CAD build for the part. Positions are in the model's coordinates, mm. Round coordinates to 2 decimals unless told otherwise and drop trailing zeros. Loops run counter-clockwise (first coordinate to the right, second up) from the corner with the lowest first, then second, coordinate; pieces in that order, holes last. Notation, with made-up numbers: M -35.5,78.5 L -10.5,78.5 A24 ccw -10.5,89.5 Z; hole C 83.5,-9.75 d3. An arc over 180 degrees is marked long. One line per item, written item: value. Start each with the question number.
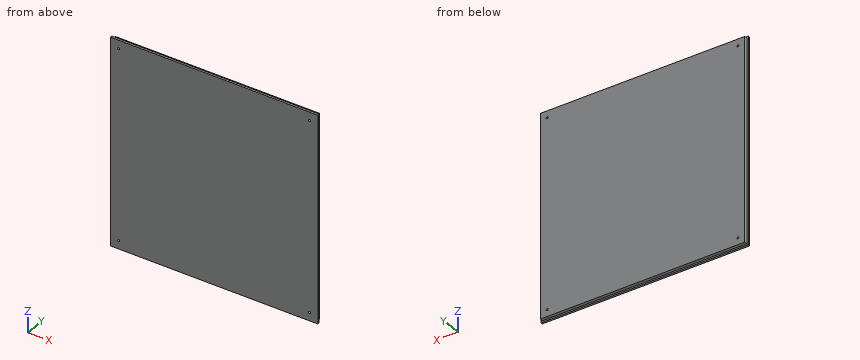
Autodesk Inventor part; units mm, degrees
ref_plane "YZ Plane" through (0, 0, 0) normal (1, 0, 0) x (0, 1, 0)
ref_plane "XZ Plane" through (0, 0, 0) normal (0, 1, 0) x (-1, 0, 0)
ref_plane "XY Plane" through (0, 0, 0) normal (0, 0, 1) x (1, 0, 0)
sketch "Boceto1" plane through (0, 0, 0) normal (0, 1, 0) x (-1, 0, 0)
  line L0 (-103, 103) -> (103, 103)
  line L1 (103, 103) -> (103, -103)
  line L2 (103, -103) -> (-103, -103)
  line L3 (-103, -103) -> (-103, 103)
  line L4 (-103, 103) -> (103, -103) construction
  line L5 (103, 103) -> (-103, -103) construction
  point P0 (0, 0)
  dimension "d0" = 206
  dimension "d1" = 206
extrude "Extrusión1" add sketch "Boceto1" along normal blind 5
sketch "Boceto3" plane through (0, 5, 0) normal (0, 1, 0) x (1, 0, 0)
  line L0 (85, 100) -> (103, 100)
  line L1 (103, -103) -> (103, 103)
  line L2 (100, -85) -> (100, 85)
  line L3 (100, 85) -> (100, 100)
  line L4 (100, 100) -> (116.202, 100) construction
  arc A0 (85, 100) -> (100, 85) centre (100, 100) ccw
  line L5 (89.3934, 89.3934) -> (89.3934, 100)
  line L6 (89.3934, 89.3934) -> (100, 89.3934)
  line L7 (89.3934, 100) -> (100, 89.3934)
  line L8 (89.3934, 89.3934) -> (100, 100)
  circle A1 centre (94.6967, 94.6967) radius 1
  circle A2 centre (-94.6967, 94.6967) radius 1
  circle A3 centre (-94.6967, -94.6967) radius 1
  circle A4 centre (94.6967, -94.6967) radius 1
  point P0 (0, 0)
  dimension "d12" = 2
  dimension "d15" = 360
hole "Agujero1" at (-94.6967, 5, -94.6967) at (-94.6967, 5, 94.6967) at (94.6967, 5, 94.6967) at (94.6967, 5, -94.6967) direction (0, -1, 0) diameter 2 end through all
sketch "Boceto4" plane through (0, 5, 0) normal (0, 1, 0) x (1, 0, 0)
  line L0 (-101.5, 101.5) -> (101.5, 101.5)
  line L1 (101.5, 101.5) -> (101.5, -101.5)
  line L2 (101.5, -101.5) -> (-101.5, -101.5)
  line L3 (-101.5, -101.5) -> (-101.5, 101.5)
  line L4 (-101.5, 101.5) -> (101.5, -101.5) construction
  line L5 (101.5, 101.5) -> (-101.5, -101.5) construction
  line L6 (-103, -103) -> (103, -103)
  line L7 (103, -103) -> (103, 103)
  line L8 (103, 103) -> (-103, 103)
  line L9 (-103, 103) -> (-103, -103)
  point P0 (0, 0)
  dimension "d24" = 203
  dimension "d25" = 203
  dimension "d26" = 206
  dimension "d27" = 206
extrude "Extrusión3" cut sketch "Boceto4" against normal blind 3
sketch "Boceto5" plane through (0, 0, 0) normal (0, -1, 0) x (1, 0, 0)
  point P0 (0, 0)
sketch "Boceto6" plane through (0, 0, 0) normal (0, -1, 0) x (1, 0, 0)
  point P0 (0, 0)
properties part number "tapa_cuboLed"
(1) Probe L1, parallel to Z at x = 55.5, y = 2.7. List the from-to ranges inside material, lowest first.
(2) Slice it at A-A, the plane y = 3.3. List the corners of the cut face in (x, z), and give its area (3 significant figures).
(3) Flat gauge pin, fed straight in: P1, Ø1.5, axis at y = 3, z = -38.5, coming from the +X side. Where does the tip first touch, or does it go through?
Check result:
1. L1: z = -101.5 to 101.5
2. outline: M -101.5,-101.5 L 101.5,-101.5 L 101.5,101.5 L -101.5,101.5 Z; hole C -94.7,-94.7 d2; hole C -94.7,94.7 d2; hole C 94.7,-94.7 d2; hole C 94.7,94.7 d2
2. area: 41,200 mm^2
3. P1: stops at x = 101.5
